from build123d import *

# Parameters (mm, degrees)
SKETCH_1_R          = 35
EXTRUDE_1_DEPTH     = 12
CUT_EXTRUDE_1_DEPTH = 4
SKETCH_3_R          = 2
CUT_EXTRUDE_2_DEPTH = 5
FILLET_1_R          = 5
SKETCH_4_R          = 20
CUT_EXTRUDE_3_DEPTH = 10
FILLET_2_R          = 5
SKETCH_5_R          = 23.6
CUT_EXTRUDE_4_DEPTH = 2.3


with BuildPart() as part:
    # 草图1 → 凸台-拉伸1 (new body)
    with BuildSketch(Plane(origin=(0, 0, 0), x_dir=(1, 0, 0), z_dir=(0, 1, 0))):
        with Locations(Location((0, 0, 0), (0, 0, 270))):
            Circle(SKETCH_1_R)
    extrude(amount=EXTRUDE_1_DEPTH)

    # 草图2 → 切除-拉伸1 (cut)
    with BuildSketch(Plane.XZ):
        Polygon((-18.2, -27.250932706), (-14.5, -29.387128702), (-10.8, -27.250932706), (-10.8, -22.978540714), (-14.5, -20.842344718), (-18.2, -22.978540714), align=None)
        Polygon((32.7, -2.136195996), (32.7, 2.136195996), (29, 4.272391992), (25.3, 2.136195996), (25.3, -2.136195996), (29, -4.272391992), align=None)
        Polygon((-14.5, 29.387128702), (-18.2, 27.250932706), (-18.2, 22.978540714), (-14.5, 20.842344718), (-10.8, 22.978540714), (-10.8, 27.250932706), align=None)
    extrude(amount=-CUT_EXTRUDE_1_DEPTH, mode=Mode.SUBTRACT)

    # 草图3 → 切除-拉伸2 (cut)
    with BuildSketch(Plane.XZ.offset(-4)):
        with Locations(Location((29, 0, 0), (0, 0, 270))):
            Circle(SKETCH_3_R)
        with Locations(Location((-14.5, -25.11473671, 0), (0, 0, 270))):
            Circle(SKETCH_3_R)
        with Locations(Location((-14.5, 25.11473671, 0), (0, 0, 270))):
            Circle(SKETCH_3_R)
    extrude(amount=-CUT_EXTRUDE_2_DEPTH, mode=Mode.SUBTRACT)

    # 圆角1
    fillet_1_edges = [part.edges().sort_by_distance(p)[0] for p in [
        (0, 12, -35),
    ]]
    fillet(fillet_1_edges, radius=FILLET_1_R)

    # 草图4 → 切除-拉伸3 (cut)
    with BuildSketch(Plane.XZ):
        with Locations(Location((0, 0, 0), (0, 0, 270))):
            Circle(SKETCH_4_R)
    extrude(amount=-CUT_EXTRUDE_3_DEPTH, mode=Mode.SUBTRACT)

    # 圆角2
    fillet_2_edges = [part.edges().sort_by_distance(p)[0] for p in [
        (0, 10, 20),
    ]]
    fillet(fillet_2_edges, radius=FILLET_2_R)

    # 草图5 → 切除-拉伸4 (cut)
    with BuildSketch(Plane.XZ):
        with Locations(Location((0, 0, 0), (0, 0, 270))):
            Circle(SKETCH_5_R)
    extrude(amount=-CUT_EXTRUDE_4_DEPTH, mode=Mode.SUBTRACT)


solid = part.part
The model under review builds one solid part; all positions refer to its coordinate system, in mm. A direction names the side the tool comes from. Coordinates: 2 decimals unless noted, no trailing zeros. Loops run counter-clockwise (first coordinate to the right, second up) from the corner with the lowest first, then second, coordinate; pieces in that order, holes last. Notation, with made-up numbers: (82, 74) -> (92, 74) arc R23 cw to (92, 109) -> close; hole circle Ø7 at (65.25, 60.25). An arc over 180 degrees is marked (long way). Use a Markdown table: item, result. Add a question column.
1. Machinability: for faces 1 (the face through (-16.38, 1.97, 21.93)), 2 (the face through (-21, 3, -28)), which of the approach directions +Z, -Z, +X, -X, +Y, -Y give a long, thin tool a straight path to every point of the face, cutting with its end or side? Answer none if there is none.
2. Add section A-A on x = 0. Write out the cut boundary in (y, z), plus the area to 3 significant figures.
3. Add section C-C on y = 6. Write out the cut boundary in (x, z), plus the area to 3 significant figures.
4. Add section B-B on z = 0. Write out the cut boundary in (x, y).
5. Clearance check with flat-ended pins moving along their axes: pin 1 Ø4.5 at (y, z) = (2.5, -0.5) entering from +X; pin 2 Ø1.2 at (x, z) = (-14.5, -24) entering from -Y; pin 3 Ø4 at (x, y) = (5.5, 4) entering from +Z. State where each tip first meets the part, or that it passes through.
6. To check wall thickness, follow line 1 (X direction, y = 1.4, z = 0); line 2 (X direction, y = 7.3, z = 0); line 3 (Y direction, x = -14, z = -6). State the ranges of each line that lie inside material, in increasing order.
Returned:
| question | item | result |
|---|---|---|
| 1 | face 1 | -Y |
| 1 | face 2 | +Y, -Y |
| 2 | outline | (0, -35) -> (7, -35) arc R5 ccw to (12, -30) -> (12, 30) arc R5 ccw to (7, 35) -> (0, 35) -> (0, 23.6) -> (2.3, 23.6) -> (2.3, 20) -> (5, 20) arc R5 cw to (10, 15) -> (10, -15) arc R5 cw to (5, -20) -> (2.3, -20) -> (2.3, -23.6) -> (0, -23.6) -> close |
| 2 | area | 423 mm² |
| 3 | outline | circle Ø70 at (0, 0); hole circle Ø39.8 at (0, 0); hole circle Ø4 at (-14.5, -25.11); hole circle Ø4 at (-14.5, 25.11); hole circle Ø4 at (29, 0) |
| 3 | area | 2,570 mm² |
| 4 | outline | (-35, 0) -> (-23.6, 0) -> (-23.6, 2.3) -> (-20, 2.3) -> (-20, 5) arc R5 cw to (-15, 10) -> (15, 10) arc R5 cw to (20, 5) -> (20, 2.3) -> (23.6, 2.3) -> (23.6, 0) -> (25.3, 0) -> (25.3, 4) -> (27, 4) -> (27, 9) -> (31, 9) -> (31, 4) -> (32.7, 4) -> (32.7, 0) -> (35, 0) -> (35, 7) arc R5 ccw to (30, 12) -> (-30, 12) arc R5 ccw to (-35, 7) -> close |
| 5 | pin 1 | stops at x = 35 |
| 5 | pin 2 | stops at y = 9 |
| 5 | pin 3 | stops at z = 34.82 |
| 6 | line 1 | x = -35 to -23.6, 23.6 to 25.3, 32.7 to 35 |
| 6 | line 2 | x = -34.99 to -19.44, 19.44 to 27, 31 to 34.99 |
| 6 | line 3 | y = 9.99 to 12 |
